Autodesk Inventor part; units mm, degrees
ref_plane "YZ Plane" through (0, 0, 0) normal (1, 0, 0) x (0, 1, 0)
ref_plane "XZ Plane" through (0, 0, 0) normal (0, 1, 0) x (-1, 0, 0)
ref_plane "XY Plane" through (0, 0, 0) normal (0, 0, 1) x (1, 0, 0)
sketch "Sketch1" plane through (0, 0, 0) normal (0, 0, 1) x (1, 0, 0)
  line L0 (25, 5.55) -> (-25, 5.55) construction
  line L1 (-25, 5.55) -> (-25, -5.55) construction
  line L2 (-25, -5.55) -> (25, -5.55) construction
  line L3 (25, -5.55) -> (25, 5.55) construction
  line L4 (25.1, -5.55) -> (25.1, 149.35) construction
  line L5 (25.1, -5.55) -> (35.1, -5.55) construction
  line L6 (35.1, -5.55) -> (35.1, 149.35) construction
  line L7 (25.1, 149.35) -> (35.1, 149.35) construction
  line L8 (25, 25.65) -> (25, 5.65)
  line L9 (25, 5.65) -> (-10, 5.65)
  line L10 (20, 25.65) -> (20, 10.65)
  line L11 (20, 10.65) -> (-10, 10.65)
  line L12 (20, 25.65) -> (25, 25.65)
  line L13 (-10, 10.65) -> (-10, 5.65)
  point P0 (0, 0)
  dimension "d0" = 0.1
  dimension "d1" = 0.1
  dimension "d2" = 5
  dimension "d3" = 35
  dimension "d4" = 20
extrude "Extrusion1" add sketch "Sketch1" against normal blind 50
sketch "Sketch2" plane through (20, 10.65, 0) normal (-1, 0, 0) x (0, 0, 1)
  circle A0 centre (-40, 7.5) radius 2.65
  line L0 (-50, 0) -> (-50, 15)
  line L1 (-50, 7.5) -> (-0.7445, 7.5) construction
  line L2 (0, 15) -> (-50, 15)
  line L3 (-25, 15) -> (-25, 0) construction
  line L4 (0, 0) -> (-50, 0)
  circle A1 centre (-10, 7.5) radius 2.65
  circle A2 centre (-25, 7.5) radius 2.65
  point P0 (0, -10.65)
  dimension "d7" = 5.3
  dimension "d8" = 10
  dimension "d9" = 5.3
extrude "Extrusion2" cut sketch "Sketch2" against normal through all
sketch "Sketch3" plane through (-10, 10.65, 0) normal (0, 1, 0) x (1, 0, 0)
  circle A0 centre (6, 10) radius 2.65
  line L0 (30, 0) -> (0, 0)
  line L1 (0, 0) -> (0, 50)
  line L2 (6, 0) -> (6, 49.4853) construction
  line L3 (0, 0) -> (0, 50)
  line L4 (0, 25) -> (30, 25) construction
  line L5 (30, 22.35) -> (30, 27.65)
  circle A1 centre (6, 40) radius 2.65
  circle A2 centre (6, 25) radius 2.65
  point P0 (10, 0)
  dimension "d12" = 5.3
  dimension "d13" = 10
  dimension "d14" = 6
  dimension "d15" = 5.3
extrude "Extrusion3" cut sketch "Sketch3" against normal through all
fillet "Fillet1" radius 2 1 edges at (20, 10.65, -25)
equation "\"d9\" = d7"
equation "\"d15\" = d12"
properties part number "Linear Rail Frame Bracket"
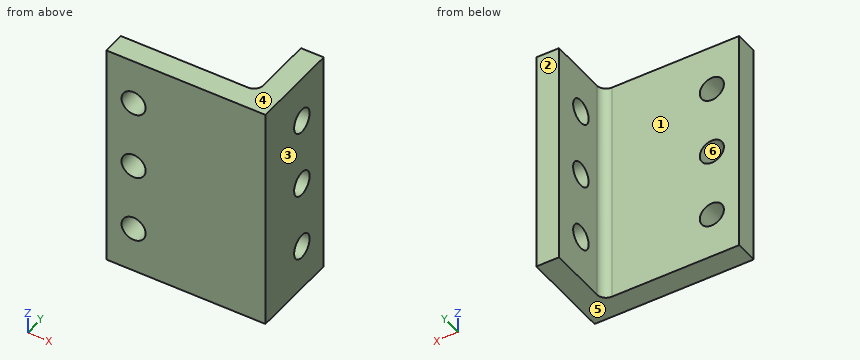
The listing builds one solid part. Answer for the finished solid, in the listing's coordinates (mm). Face numbers are marked on the shaded views. A direction names the side the tool comes from. Coordinates: 2 decimals unless noted, no trailing zeros. Loops run counter-clockwise (first coordinate to the right, second up) from the corner with the lowest first, then second, coordinate; pieces in that order, holes last. Notation, with made-up numbers: (17, 7) - (55, 7) arc R17 cw to (55, 19) - close; hole circle Ø5 at (-4, 40). An arc over 180 degrees is marked (long way). Use a Markdown table: item, result. Add a question column.
1) Find the intervals of material crossed by line 1 (X direction, y = 7.9, z = -10); line 2 (Y direction, x = 21.4, z = -40); line 3 (Z direction, x = -4, y = 7.35), in increasing order.
2) The part is cut by section D-D, the plane z = -32.5. Give the vertices of the cut face in (x, y), and give its area (3 significant figures).
3) The part is cut by section A-A, the plane x = -4. Give the vertices of the cut face in (y, z), and give its area (4 significant figures).
4) The part is cut by section B-B, the plane y = 18.15. Give the vertices of the cut face in (x, z), and give its area (4 significant figures).
5) Given pin 1 (5 mm diameter, centred on x = -2, y = 11.5, fed in from -Z); pin 2 (10 mm diameter, centred on x = -4, z = -19, fed in from +Y); pin 3 (1 mm diameter, centred on y = 14.5, z = -39, fed in from -X), each flat-ended and moving along its own axis, determine where each tip first touches the part or whether it passes through.
6) For the marked faces 1 and 2, determine the directions among +Z, -Z, +X, -X, +Y, -Y from which every point of the face is accessible in a straight line to the end or side of a thin tool.
7) The mould has two halves that part along Z. Classify the marked faces 3, 4, 5 and 6: released by +Z, released by -Z, zero draft, split by the parting line, or undercut.
8) The part is cut by section C-C, the plane z = -25. Give the vertices of the cut face in (x, y).
Here are the results:
| question | item | result |
|---|---|---|
| 1 | line 1 | x = -10 to -6.65, -1.35 to 25 |
| 1 | line 2 | y = 5.65 to 15.5, 20.8 to 25.65 |
| 1 | line 3 | z = -50 to -42.65, -37.35 to -27.65, -22.35 to -12.65, -7.35 to 0 |
| 2 | outline | (-10, 5.65) - (25, 5.65) - (25, 25.65) - (20, 25.65) - (20, 12.65) arc R2 cw to (18, 10.65) - (-10, 10.65) - close |
| 2 | area | 251 mm^2 |
| 3 | outline | (5.65, -50) - (10.65, -50) - (10.65, -42.65) - (5.65, -42.65) - close; (5.65, -37.35) - (10.65, -37.35) - (10.65, -27.65) - (5.65, -27.65) - close; (5.65, -22.35) - (10.65, -22.35) - (10.65, -12.65) - (5.65, -12.65) - close; (5.65, -7.35) - (10.65, -7.35) - (10.65, 0) - (5.65, 0) - close |
| 3 | area | 170.5 mm^2 |
| 4 | outline | (20, -50) - (25, -50) - (25, -42.65) - (20, -42.65) - close; (20, -37.35) - (25, -37.35) - (25, -27.65) - (20, -27.65) - close; (20, -22.35) - (25, -22.35) - (25, -12.65) - (20, -12.65) - close; (20, -7.35) - (25, -7.35) - (25, 0) - (20, 0) - close |
| 4 | area | 170.5 mm^2 |
| 5 | pin 1 | stops at z = -50 |
| 5 | pin 2 | stops at y = 10.65 |
| 5 | pin 3 | stops at x = 20 |
| 6 | face 1 | +Z, -Z, -X, +Y |
| 6 | face 2 | +Z, -Z, +X, -X, +Y |
| 7 | face 3 | zero draft |
| 7 | face 4 | released by +Z |
| 7 | face 5 | released by -Z |
| 7 | face 6 | undercut |
| 8 | outline | (-10, 5.65) - (-6.65, 5.65) - (-6.65, 10.65) - (-10, 10.65) - close; (-1.35, 5.65) - (25, 5.65) - (25, 15.5) - (20, 15.5) - (20, 12.65) arc R2 cw to (18, 10.65) - (-1.35, 10.65) - close; (20, 20.8) - (25, 20.8) - (25, 25.65) - (20, 25.65) - close |
